```python
from build123d import *

# Parameters (mm, degrees)
SKETCH_4_R          = 3
SKETCH_4_W          = 50
SKETCH_4_H          = 3
EXTRUDE_1_DEPTH     = 3
SKETCH_5_R          = 1.5
CUT_EXTRUDE_1_DEPTH = 1.2
SKETCH_6_R          = 0.6
CUT_EXTRUDE_2_DEPTH = 29.319604517


with BuildPart() as part:
    # 草图4 → 凸台-拉伸1 (new body)
    with BuildSketch(Plane(origin=(0, 0, 0), x_dir=(1, 0, 0), z_dir=(0, 1, 0))):
        Circle(SKETCH_4_R)
        with Locations((25, 0)):
            Circle(SKETCH_4_R)
        with Locations((-25, 0)):
            Circle(SKETCH_4_R)
        Rectangle(SKETCH_4_W, SKETCH_4_H)
    extrude(amount=EXTRUDE_1_DEPTH)

    # 草图5 → 切除-拉伸1 (cut)
    with BuildSketch(Plane.XZ):
        with Locations(Location((-25, 0, 0), (0, 0, 270))):
            Circle(SKETCH_5_R)
        with Locations(Location((0, 0, 0), (0, 0, 270))):
            Circle(SKETCH_5_R)
        with Locations(Location((25, 0, 0), (0, 0, 270))):
            Circle(SKETCH_5_R)
    extrude(amount=-CUT_EXTRUDE_1_DEPTH, mode=Mode.SUBTRACT)

    # 草图6 → 切除-拉伸2 (cut, through all)
    with BuildSketch(Plane(origin=(0, 0, 0), x_dir=(-1, 0, 0), z_dir=(0, -1, 0))):
        with Locations(Location((0, 0, 0), (0, 0, 90))):
            Circle(SKETCH_6_R)
        with Locations(Location((-25, 0, 0), (0, 0, 90))):
            Circle(SKETCH_6_R)
        with Locations(Location((25, 0, 0), (0, 0, 90))):
            Circle(SKETCH_6_R)
    extrude(amount=-CUT_EXTRUDE_2_DEPTH, mode=Mode.SUBTRACT)


solid = part.part
```
Could you check a few things on this model? Use its own coordinates, in mm. A direction names the side the tool comes from. Coordinates: 2 decimals unless noted, no trailing zeros. Order: outer loops, then holes, each group sorted by start corner. A loop starts at its lowest first (then second) coordinate and runs counter-clockwise, first axis right, second up. Notation, with made-up numbers: M -11,46.25 L 7,46.25 A11 ccw 7,51.25 Z; hole C 35,88 d7. An arc over 180 degrees is marked long. Use one line per item in the form item = value. Start each with the question number.
1. Suppose I cut it at D-D on z = 2.35. Write out the boundary of the cut face in (x, y), then the cut area to 3 significant figures.
2. Suppose I cut it at B-B on x = -25. Write out the boundary of the cut face in (y, z).
3. For pin 1 (1.5 mm diameter, centred on y = 0.5, z = 1, fed in from +X); pin 2 (1.5 mm diameter, centred on x = -9, y = 1, fed in from -Z); pin 3 (1.4 mm diameter, centred on x = 0, z = 0, fed in from -Y), each with a flat end and sliding along its axis, tell me the tip position at first contact or that it passes through.
4. Suppose I cut it at A-A on z = 0. Write out the boundary of the cut face in (x, y).
5. On a 3-axis mill with a long thin cutter (end or side, diameter ignored), from which of +Z, -Z, +X, -X, +Y, -Y can I reach the whole of each face in a straight line? I mean faces 1 (the flat face through (-13, 1, -1.5)), 2 (the flat face through (-25, 1.2, -1)), 3 (the flat face through (12, 1, 1.5)). Say none if no direction works.
6. Suppose I cut it at C-C on y = 2. Write out the boundary of the cut face in (x, z), then the cut area to 3 significant figures.
7. Please list where these lines run through material, in increasing order: line 1 (X direction, y = 2.45, z = 0); line 2 (X direction, y = 0.5, z = 0); line 3 (Z direction, x = 19.5, y = 0.7).
8. We'd pull the mould along Z, two halves only. Please class faces 4 (the flat face through (25, 1.2, -1)), 5 (the cylindrical face through (-28, 1, 0)), 6 (the flat face through (12, 1, -1.5)): +Z half, -Z half, draft (parallel to the pull), parting line (faces both ways), or undercut.
Geometry says:
q1.outline = M -26.86,0 L -23.14,0 L -23.14,3 L -26.86,3 Z; M -1.86,0 L 1.86,0 L 1.86,3 L -1.86,3 Z; M 23.14,0 L 26.86,0 L 26.86,3 L 23.14,3 Z
q1.area = 33.6 mm^2
q2.outline = M 0,-3 L 3,-3 L 3,-0.6 L 1.2,-0.6 L 1.2,-1.5 L 0,-1.5 Z; M 0,1.5 L 1.2,1.5 L 1.2,0.6 L 3,0.6 L 3,3 L 0,3 Z
q3.pin_1 = 27.99
q3.pin_2 = -1.5
q3.pin_3 = 1.2
q4.outline = M -28,0 L -26.5,0 L -26.5,1.2 L -25.6,1.2 L -25.6,3 L -28,3 Z; M -24.4,1.2 L -23.5,1.2 L -23.5,0 L -1.5,0 L -1.5,1.2 L -0.6,1.2 L -0.6,3 L -24.4,3 Z; M 0.6,1.2 L 1.5,1.2 L 1.5,0 L 23.5,0 L 23.5,1.2 L 24.4,1.2 L 24.4,3 L 0.6,3 Z; M 25.6,1.2 L 26.5,1.2 L 26.5,0 L 28,0 L 28,3 L 25.6,3 Z
q5.face_1 = -Z, +Y, -Y
q5.face_2 = -Y
q5.face_3 = +Z, +Y, -Y
q6.outline = M -22.4,-1.5 L -2.6,-1.5 A3 ccw 2.6,-1.5 L 22.4,-1.5 A3 ccw long 22.4,1.5 L 2.6,1.5 A3 ccw -2.6,1.5 L -22.4,1.5 A3 ccw long Z; hole C -25,0 d1.2; hole C 0,0 d1.2; hole C 25,0 d1.2
q6.area = 197 mm^2
q7.line_1 = -28 to -25.6, -24.4 to -0.6, 0.6 to 24.4, 25.6 to 28
q7.line_2 = -28 to -26.5, -23.5 to -1.5, 1.5 to 23.5, 26.5 to 28
q7.line_3 = -1.5 to 1.5
q8.face_4 = undercut
q8.face_5 = parting line
q8.face_6 = -Z half
